Design review of the part built by this model. Coordinates are the model's own, in mm. Coordinates: 2 decimals unless noted, no trailing zeros. Write each loop counter-clockwise with the first axis right and the second up, starting at its lowest first coordinate (ties: lowest second). Pieces come first, ordered by that corner, then holes. Notation, with made-up numbers: (51, -19.5) -> (100, -19.5) arc R15 ccw to (100, 0.5) -> close; hole circle Ø4 at (-2.75, 73.25). An arc over 180 degrees is marked (long way). Return JSON: item names as keys, results as strings. Group by question number.
from build123d import *

# Parameters (mm, degrees)
F1_DEPTH = 45
F2_R     = 0.6


with BuildPart() as f1:
    # F0 (on Front) → F1 (new body)
    with BuildSketch(Plane.XZ):
        Polygon((2.034771, 4.105063), (2.432787, 0.124914), (8.432787, 0.126559), (6.01492, 4.503078), align=None)
    extrude(amount=F1_DEPTH)

    # F2
    f2_edges = [f1.edges().sort_by_distance(p)[0] for p in [
        (2.034771, -22.5, 4.105063),
        (6.01492, -22.5, 4.503078),
    ]]
    fillet(f2_edges, radius=F2_R)


solid = f1.part
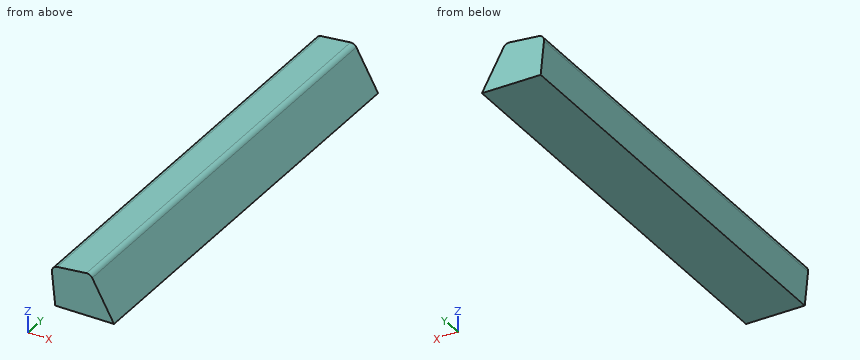
Q1. We need section C-C on z = 1.9. Write out the cut boundary in (x, y).
Q2. Wall thickness on L1, parallel to Z at x = 4, y = -31; L2, parallel to X at y = -27.5, z = 3.6; L3, parallel to X at y = -12, z = 1.2: over which ranges is each line inside the solid? List them lowest first.
Q3. We need section A-A on y = -25.5. Write out the cut boundary in (x, z).
Q4. We need section B-B on x = 4.25. Write out the cut boundary in (y, z), plus the area to 3 significant figures.
Q5. For P1, Ø1.5, axis at x = 7, y = -35.5, coming from the +Z side, flat-tipped, find the tip position at first contact; note if it passes through.
Findings below:
{
 "1": {"outline": "(2.26, -45) -> (7.45, -45) -> (7.45, 0) -> (2.26, 0) -> close"},
 "2": {"L1": "z = 0.13 to 4.3", "L2": "x = 2.09 to 6.51", "L3": "x = 2.33 to 7.84"},
 "3": {"outline": "(2.09, 3.51) -> (2.43, 0.12) -> (8.43, 0.13) -> (6.21, 4.16) arc R0.6 ccw to (5.62, 4.46) -> (2.63, 4.16) arc R0.6 ccw to start"},
 "4": {"outline": "(-45, 0.13) -> (0, 0.13) -> (0, 4.33) -> (-45, 4.33) -> close", "area": "189 mm^2"},
 "5": {"P1": "stops at z = 4.08"}
}
